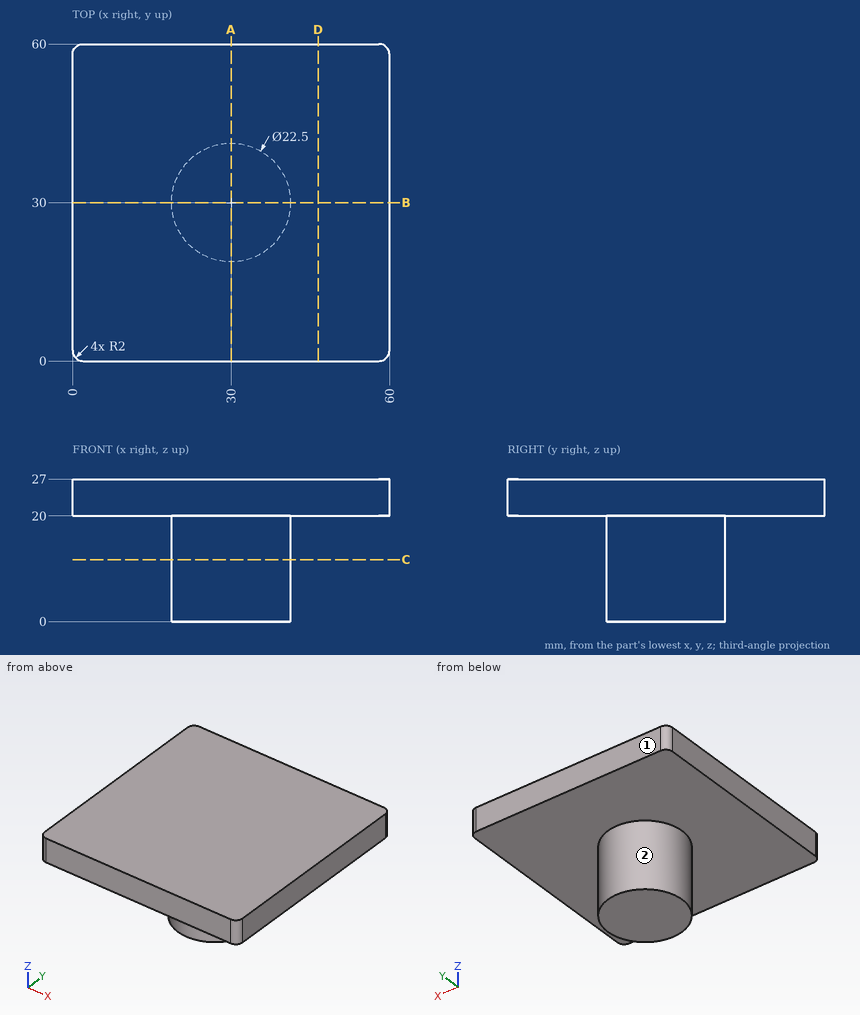
Part print with two shaded views. Sizes in mm from the minimum x, y, z corner. A direction names the side the tool comes from. Round coordinates to 2 decimals unless told otherwise and drop trailing zeros. Write each loop counter-clockwise with the first axis right and the second up, starting at its lowest first coordinate (ties: lowest second). Pieces come first, ordered by that corner, then holes. Notation, with made-up numbers: M -30,-27.5 L -16,-27.5 A6 ccw -16,-19.5 Z; hole C 9,44 d7. An arc over 180 degrees is marked long. Use CSV: the item, a comma, the result in double quotes.
1. Wall check: probe 1 along Z at (x, y) = (49.5, 15.5); probe 2 along X at (y, z) = (31, 14.75). Give the ranges that are in metal, low to high. Write a range as from..to.
Reply:
probe 1,"z = 20..27"
probe 2,"x = 18.79..41.21"
2. Saw through at A-A (x = 30). Give the cut face in (y, z).
Reply:
outline,"M 0,20 L 18.75,20 L 18.75,0 L 41.25,0 L 41.25,20 L 60,20 L 60,27 L 0,27 Z"
3. Saw through at C-C (z = 11.75). Give the cut face in (x, y), plus the area to 3 significant figures.
Reply:
outline,"C 30,30 d22.5"
area,"398 mm²"
4. Flat gauge pins, fed straight in: pin 1 (2 mm diameter, centred on x = 16.5, z = 3.5, fed in from +Y); pin 2 (4 mm diameter, centred on x = 26, y = 51.5, fed in from -Z). Where does each tip first touch, or does it go through?
Reply:
pin 1,"passes through"
pin 2,"stops at z = 20"
5. Saw through at D-D (x = 46.5). Give the cut face in (y, z).
Reply:
outline,"M 0,20 L 60,20 L 60,27 L 0,27 Z"
6. Tool access for the marked faces 1 and 2: list every direction of +Z, -Z, +X, -X, +Y, -Y with a clear straight run to the whole face (end or side of a thin tool).
Reply:
face 1,"+Z, -Z, +X, -X, +Y"
face 2,"-Z"
